Here's how the part is built. I have some questions about the finished solid (model axes, mm). Face numbers are marked on the shaded views. A direction names the side the tool comes from. Coordinates: 2 decimals unless noted, no trailing zeros. Loops run counter-clockwise (first coordinate to the right, second up) from the corner with the lowest first, then second, coordinate; pieces in that order, holes last. Notation, with made-up numbers: (-24, -12.5) - (27, -12.5) arc R19 cw to (27, -7.5) - close; hole circle Ø1 at (32, 31.5). An arc over 180 degrees is marked (long way). Use a Markdown table: item, result.
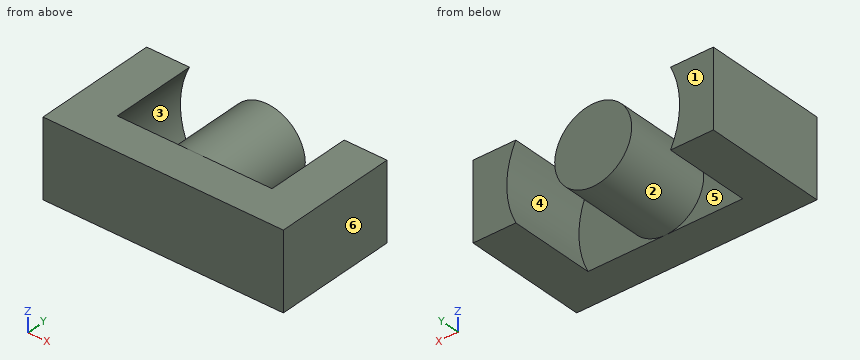
```python
from build123d import *

# Parameters (mm, degrees)
SKETCH1_W          = 30.6
SKETCH1_H          = 9.8
BASE_EXTRUDE_DEPTH = 15.8
SKETCH2_R          = 11
SKETCH2_R_2        = 4.9
CUT_EXTRUDE1_DEPTH = 11


with BuildPart() as part:
    # Sketch1 → Base-Extrude (new body)
    with BuildSketch(Plane(origin=(0, 0, 0), x_dir=(1, 0, 0), z_dir=(0, 1, 0))):
        Rectangle(SKETCH1_W, SKETCH1_H)
    extrude(amount=BASE_EXTRUDE_DEPTH)

    # Sketch2 → Cut-Extrude1 (cut)
    with BuildSketch(Plane(origin=(0, 15.8, 0), x_dir=(-1, 0, 0), z_dir=(0, 1, 0))):
        Circle(SKETCH2_R)
        with Locations(Location((0, 0, 0), (0, 0, 90))):
            Circle(SKETCH2_R_2, mode=Mode.SUBTRACT)
    extrude(amount=-CUT_EXTRUDE1_DEPTH, mode=Mode.SUBTRACT)


solid = part.part
```
Q1. Please list where these lines run through material, in increasing order: L1, parallel to X at y = 11.75, z = 0.25; L2, parallel to X at y = 13, z = -2.25; L3, parallel to Y at x = 6, z = 2.25. Write a range as from..to.
Check values:
| item | result |
|---|---|
| L1 | -15.3..-11, -4.89..4.89, 11..15.3 |
| L2 | -15.3..-10.77, -4.35..4.35, 10.77..15.3 |
| L3 | 0..4.8 |
Q2. I want a section at D-D, the plane z = -3.5. Write out the boundary of the cut face in (x, y).
Check values:
| item | result |
|---|---|
| outline | (-15.3, 0) - (15.3, 0) - (15.3, 15.8) - (10.43, 15.8) - (10.43, 4.8) - (3.43, 4.8) - (3.43, 15.8) - (-3.43, 15.8) - (-3.43, 4.8) - (-10.43, 4.8) - (-10.43, 15.8) - (-15.3, 15.8) - close |
Q3. Which directions (+Z, -Z, +X, -X, +Y, -Y) give clear straight access to the entire face, cutting with the end or side of a thin tool? Please do the marked faces 5 and 6.
Check values:
| item | result |
|---|---|
| face 5 | +Y |
| face 6 | +Z, -Z, +X, +Y, -Y |
Q4. I want a section at C-C, the plane x = 4.5. Write out the boundary of the cut face in (y, z).
Check values:
| item | result |
|---|---|
| outline | (0, -4.9) - (4.8, -4.9) - (4.8, -1.94) - (15.8, -1.94) - (15.8, 1.94) - (4.8, 1.94) - (4.8, 4.9) - (0, 4.9) - close |
Q5. I want a section at A-A, the plane y = 14. Write out the boundary of the cut face in (x, z), then the cut area to 3 significant figures.
Check values:
| item | result |
|---|---|
| outline | (-15.3, -4.9) - (-9.85, -4.9) arc R11 cw to (-9.85, 4.9) - (-15.3, 4.9) - close; circle Ø9.8 at (0, 0); (9.85, -4.9) - (15.3, -4.9) - (15.3, 4.9) - (9.85, 4.9) arc R11 cw to start |
| area | 167 mm^2 |
Q6. I want a section at B-B, the plane z = 0. Write out the boundary of the cut face in (x, y), then the cut area to 3 significant figures.
Check values:
| item | result |
|---|---|
| outline | (-15.3, 0) - (15.3, 0) - (15.3, 15.8) - (11, 15.8) - (11, 4.8) - (4.9, 4.8) - (4.9, 15.8) - (-4.9, 15.8) - (-4.9, 4.8) - (-11, 4.8) - (-11, 15.8) - (-15.3, 15.8) - close |
| area | 349 mm^2 |
Q7. If we mould it in two halves opening along Z, with no side actions, what happens to the marked faces 1, 2, 3 and 4? For each: pulls with the +Z half, pulls with the -Z half, needs draft (parallel to the pull), parting line crosses it, or undercut.
Check values:
| item | result |
|---|---|
| face 1 | needs draft |
| face 2 | parting line crosses it |
| face 3 | undercut |
| face 4 | undercut |
